Here's how the part is built. I have some questions about the finished solid (model axes, mm). A direction names the side the tool comes from. Coordinates: 2 decimals unless noted, no trailing zeros. Write each loop counter-clockwise with the first axis right and the second up, starting at its lowest first coordinate (ties: lowest second). Pieces come first, ordered by that corner, then holes. Notation, with made-up numbers: M -5,40 L 6,40 A19 cw 6,68 Z; hole C 31,85.5 d11. An arc over 180 degrees is marked long. Use a Markdown table: item, result.
Autodesk Fusion 360 part; units mm, degrees
sketch "Sketch1" plane through (0, 0, 0) normal (0, 1, 0) x (1, 0, 0)
  line L0 (0, 0) -> (0, -70)
  line L1 (0, 0) -> (-17.5, 0)
  spline S0 degree 5 poles (-17.5, 0) (-17.5, -1.949) (-17.4812, -5.4749) (-17.3967, -9.6483) (-17.034, -13.32) (-15.2217, -16.0242) (-11.5143, -17.5778) (-6.6893, -18.7492) (-2.4074, -19.5755) (0, -20) knots 0 0 0 0 0 0 0.2 0.4 0.6 0.8 1 1 1 1 1 1
  line L2 (-5, -19.1184) -> (5, -20.8816)
  line L3 (-17.5, 4) -> (-17.5, -4)
  line L4 (-15.4223, 0) -> (-10.3547, -57.9233)
  spline S1 degree 5 poles (-10.3547, -57.9233) (-10.6938, -58.2624) (-11.3394, -58.9222) (-12.2103, -59.8566) (-13.1936, -61.0089) (-14.1589, -62.3571) (-14.7035, -63.4078) (-14.9524, -64.1982) (-15.0388, -64.7286) (-15.0621, -64.9946) knots 0 0 0 0 0 0 0.2 0.4 0.6 0.8 1 1 1 1 1 1
  line L5 (-15.0621, -64.9946) -> (-15.5, -70)
  line L6 (-14.9783, -64.0369) -> (-15.1459, -65.9522)
  line L7 (-17.5, -70) -> (0, -70) construction
  line L8 (-15.5, -70) -> (-9.7348, -70)
  line L9 (-9.7348, -70) -> (-9.7348, -67.5)
  line L10 (-9.0716, -56.6402) -> (-11.6378, -59.2064)
  line L11 (-17.5, 0) -> (-17.5, -70) construction
  spline S2 degree 5 poles (-9.7348, -67.5) (-9.5938, -67.5) (-9.3202, -67.5511) (-8.9352, -67.7806) (-8.3991, -68.3325) (-7.2315, -69.1675) (-5.359, -69.7194) (-3.0799, -69.9489) (-1.103, -70) (0, -70) knots 0 0 0 0 0 0 0.2 0.4 0.6 0.8 1 1 1 1 1 1
  line L12 (-10.1589, -67.5) -> (-9.3107, -67.5)
  line L13 (-3.3162, -70) -> (3.3162, -70)
  line L14 (-10.3504, -57.9716) -> (-11.575, -57.6845)
  line L15 (-12.1293, -56.3884) -> (-10.6186, -54.9071)
  line L16 (-11.575, -57.6845) -> (-12.1293, -56.3884)
  dimension "d1" = 70
  dimension "d2" = 17.5
  dimension "d3" = 5
  dimension "d4" = 45
  dimension "d5" = 5
  dimension "d6" = 10
  dimension "d14" = 2.5
  dimension "d15" = 2
revolve "Revolve1" add sketch "Sketch1" angle 360 about axis through (0, 0, 0) along (0, 0, 1)
sketch "Sketch3" plane through (0, 0, 70) normal (0, 0, 1) x (-1, 0, 0)
  circle A0 centre (0, 0) radius 9.7348
  circle A1 centre (0, 0) radius 15.5
  line L0 (0, 0) -> (0.6761, -15.4852)
  line L1 (0, 0) -> (-0.6761, -15.4852)
  line L2 (0, 0) -> (0, -15.5) construction
  dimension "d8" = 5
  dimension "d9" = 2.5
extrude "Extrude1" cut sketch "Sketch3" against normal up to surface (2.5 mm away) contours A0 A1 L0 L1 picked at (0.4421, -13.5697)
pattern_circular "C-Pattern1" count 5 over 360 about axis through (0, 0, 1.75) along (0, 0, 1) of "Extrude1"
equation "d2 = 3.5 cm / 2"
1. I need wall thicknesses on probe 1 along Y at (x, z) = (-12, 15); probe 2 along X at (y, z) = (-4, 19.5); probe 3 along X at (y, z) = (-5.5, 18). Which ranges of each line are inside material? Lowest first, please.
Answers follow:
| item | result |
|---|---|
| probe 1 | y = -9.75 to 9.75 |
| probe 2 | x = -13.12 to 13.12 |
| probe 3 | x = -12.71 to 12.71 |
2. Suppose I cut it at B-B on z = 45.5. Write out the boundary of the cut face in (x, y).
Answers follow:
| item | result |
|---|---|
| outline | C 0,0 d22.88 |
3. Which directions (+Z, -Z, +X, -X, +Y, -Y) give clear straight access to the entire face, cutting with the end or side of a thin tool? Please do faces 4 (the face through (-12, 4, 67.5)), 5 (the face through (0, -12, 70)).
Answers follow:
| item | result |
|---|---|
| face 4 | +Z |
| face 5 | +Z, +X, -X, +Y, -Y |
4. We'd pull the mould along Y, two halves only. Please class faces 1 (the face through (8, 9, 70)), 2 (the face through (-7.829, -9.843, 68.768)), 3 (the face through (9.79, -7.51, 35.26)): +Y half, -Y half, draft (parallel to the pull), parting line (faces both ways), or undercut.
Answers follow:
| item | result |
|---|---|
| face 1 | draft |
| face 2 | undercut |
| face 3 | parting line |
5. Will these pins go through, and if not, where does the flat tip stop? pin 1 Ø8 at (y, z) = (12.5, 12.5) entering from -X; pin 2 Ø3 at (y, z) = (-1.5, 27) entering from +X; pin 3 Ø5 at (y, z) = (9.5, 51.5) entering from -X.
Answers follow:
| item | result |
|---|---|
| pin 1 | stops at x = -14.68 |
| pin 2 | stops at x = 13.15 |
| pin 3 | stops at x = -8.4 |
6. Suppose I cut it at A-A on z = 26.5. Write out the boundary of the cut face in (x, y), and give its area (3 significant figures).
Answers follow:
| item | result |
|---|---|
| outline | C 0,0 d26.21 |
| area | 539 mm2 |
